from build123d import *

# Parameters (mm, degrees)
SKETCH2_W               = 38.1
SKETCH2_H               = 41.6052
SKETCH2_W_2             = 33.02
SKETCH2_H_2             = 33.9852
BOSS_EXTRUDE1_DEPTH     = 5.08
BOSS_EXTRUDE2_DEPTH     = 7.62
M2_CLEARANCE_HOLE1_D    = 2.4
SKETCH8_W               = 38.1
SKETCH8_H               = 41.6052
SKETCH8_R               = 6.604
BOSS_EXTRUDE3_DEPTH     = 2.54
SKETCH7_R               = 1.50114
CUT_EXTRUDE1_DEPTH      = 3.54
CUT_EXTRUDE1_DEPTH_BACK = 13.7


with BuildPart() as part:
    # Sketch2 → Boss-Extrude1 (new body)
    with BuildSketch(Plane.XY):
        with Locations((0, 20.8026)):
            Rectangle(SKETCH2_W, SKETCH2_H)
        with Locations((0, 19.5326)):
            Rectangle(SKETCH2_W_2, SKETCH2_H_2, mode=Mode.SUBTRACT)
    extrude(amount=BOSS_EXTRUDE1_DEPTH)

    # Sketch4 → Boss-Extrude2 (add)
    with BuildSketch(Plane(origin=(0, 0, 0), x_dir=(-1, 0, 0), z_dir=(0, 0, -1))):
        Polygon((-19.05, 41.6052), (19.05, 41.6052), (19.05, 39.0652), (-19.05, 39.036199263), align=None)
    extrude(amount=BOSS_EXTRUDE2_DEPTH)

    # M2 Clearance Hole1 (through all)
    with Locations(Plane(origin=(0, 41.6052, 0), x_dir=(1, 0, 0), z_dir=(0, 1, 0))):
        with Locations((-13.97, 5.08), (13.97, 5.08)):
            Hole(M2_CLEARANCE_HOLE1_D / 2)

    # Sketch8 → Boss-Extrude3 (add)
    with BuildSketch(Plane.XY.offset(5.08)):
        with Locations((0, 20.8026)):
            Rectangle(SKETCH8_W, SKETCH8_H)
        with Locations((0, 11.02614)):
            Circle(SKETCH8_R, mode=Mode.SUBTRACT)
    extrude(amount=BOSS_EXTRUDE3_DEPTH)

    # Sketch7 → Cut-Extrude1 (cut, two sides)
    with BuildSketch(Plane.XY.offset(5.08)) as cut_extrude1_sk:
        with Locations((-10.31494, 5.715)):
            Circle(SKETCH7_R)
        with Locations((10.31494, 5.715)):
            Circle(SKETCH7_R)
    extrude(amount=CUT_EXTRUDE1_DEPTH, mode=Mode.SUBTRACT)
    extrude(cut_extrude1_sk.sketch, amount=-CUT_EXTRUDE1_DEPTH_BACK, mode=Mode.SUBTRACT)


solid = part.part
Model file for the job. Use its own axes, mm. A direction names the side the tool comes from. Round coordinates to 2 decimals unless told otherwise and drop trailing zeros. Order: outer loops, then holes, each group sorted by start corner. A loop starts at its lowest first (then second) coordinate and runs counter-clockwise, first axis right, second up. Notation, with made-up numbers: M 31.25,-33.75 L 45.25,-33.75 A31 ccw 45.25,-3.75 Z; hole C -31.5,48.5 d9. An arc over 180 degrees is marked long. Write each question's results on one line, items separated by ' | '. Start each with the question number.
(1) Probe probe 1 along X at (y, z) = (40.15, -5.08); probe 2 along Z at (x, y) = (-13.97, 40.6); probe 3 along X at (y, z) = (6, 2). List the from-to ranges inside material, lowest first. Write a range as from..to.
(2) Saw through at A-A, the plane z = 1.25. Give the cut face in (x, y), then the cut area to 3 significant figures.
(3) Saw through at D-D, the plane y = 20.5. Give the cut face in (x, z), then the cut area to 3 significant figures.
(4) Drop flat-ended pins along their axis: pin 1 (19 mm diameter, centred on x = -2, y = 24.5, fed in from -Z); pin 2 (2.5 mm diameter, centred on x = 10.31, y = 5.72, fed in from +Z); pin 3 (3 mm diameter, centred on x = 13.97, z = -5.08, fed in from -Y). Give the stop position or say it passes through.
(5) Two-plate mould, pull along Z, no slides. Class faces 1 (the face through (0, 40, -7.62)), 2 (the face through (-0.86, 17.574, 6.332)), 3 (the face through (15.17, 40.3, -5.13)): pulls with the +Z half, pulls with the -Z half, needs draft (parallel to the pull), parting line crosses it, or undercut.
(6) Which spindle directions (+Z, -Z, +X, -X, +Y, -Y) get a long thin tool onto all of the face, cutting with end or side? Do faces 4 (the face through (16.51, 19, 3)), 5 (the face through (19.05, 21, 3)). Say none if no direction does.
(7) Saw through at B-B, the plane x = 13.97. Give the cut face in (y, z), then the cut area to 3 significant figures.
(8) Saw through at C-C, the plane z = -5.75. Give the cut face in (x, y).
Established:
1) probe 1: x = -19.05..-15.17, -12.77..12.77, 15.17..19.05 | probe 2: z = -7.62..-6.28, -3.88..7.62 | probe 3: x = -19.05..-16.51, 16.51..19.05
2) outline: M -19.05,0 L 19.05,0 L 19.05,41.61 L -19.05,41.61 Z; hole M -16.51,2.54 L 16.51,2.54 L 16.51,36.53 L -16.51,36.53 Z | area: 463 mm^2
3) outline: M -19.05,0 L -16.51,0 L -16.51,5.08 L 16.51,5.08 L 16.51,0 L 19.05,0 L 19.05,7.62 L -19.05,7.62 Z | area: 123 mm^2
4) pin 1: stops at z = 5.08 | pin 2: passes through | pin 3: stops at y = 39.04
5) face 1: pulls with the -Z half | face 2: needs draft | face 3: undercut
6) face 4: -Z | face 5: +Z, -Z, +X, +Y, -Y
7) outline: M 0,0 L 2.54,0 L 2.54,5.08 L 36.53,5.08 L 36.53,0 L 39.04,0 L 39.04,-3.88 L 41.61,-3.88 L 41.61,7.62 L 0,7.62 Z; M 39.04,-7.62 L 41.61,-7.62 L 41.61,-6.28 L 39.04,-6.28 Z | area: 158 mm^2
8) outline: M -19.05,39.07 L -14.97,39.06 L -14.97,41.61 L -19.05,41.61 Z; M -12.97,39.06 L 12.97,39.04 L 12.97,41.61 L -12.97,41.61 Z; M 14.97,39.04 L 19.05,39.04 L 19.05,41.61 L 14.97,41.61 Z
